Check sheet for the modelled part. Datum: model origin and axes. Units: mm. Face numbers are marked on the shaded views. Give positions to 0.01 mm unless a question says otherwise; leave off trailing zeros. Loops run counter-clockwise (first coordinate to the right, second up) from the corner with the lowest first, then second, coordinate; pieces in that order, holes last. Notation, with made-up numbers: M 30,57 L 49,57 A16 ccw 49,63 Z; hole C 12.5,57 d7. An arc over 180 degrees is marked long. Write each question's results on one line, items separated by ' | '. Start each with the question number.
1. Sectioned sample at B-B on y = 14.25. Record the cut outline in (x, z).
2. Sectioned sample at C-C on x = -14.75. Record the cut outline in (y, z).
3. Go/stop test with flat-tipped pins: pin 1 (2.5 mm diameter, centred on y = 11.88, z = -7, fed in from -X); pin 2 (5 mm diameter, centred on y = 11.88, z = -7, fed in from -X); pin 3 (5 mm diameter, centred on y = 16, z = -4, fed in from +X); pin 4 (4 mm diameter, centred on x = -12, z = -9, fed in from +Y). Record where each tip stops, or that it passes through.
4. Sectioned sample at A-A on x = -9.5. Record the cut outline in (y, z), and give its area (3 significant figures).
5. Material ranges on line 1 along Z through (x, y) = (-15.75, 10.5); line 2 along Y through (x, z) = (-4.45, -7); line 3 along Y through (x, z) = (-14.65, 7), recorded low to high.
6. Draft check along X on the marked faces 1, 2 and 3. Enter one of: pulls with the +X half, pulls with the -X half, needs draft (parallel to the pull), parting line crosses it, or undercut.
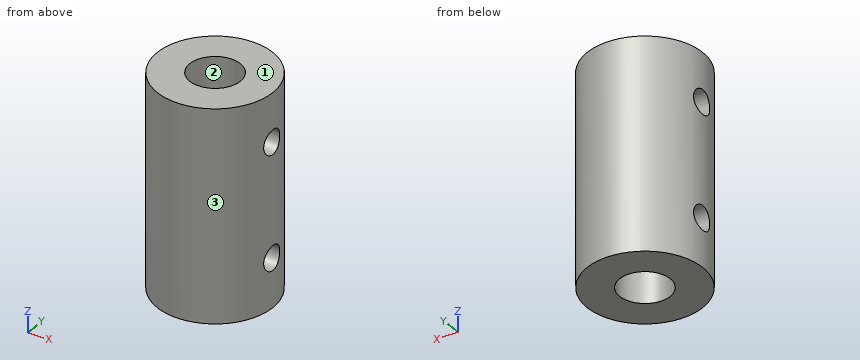
```python
from build123d import *

# Parameters (mm, degrees)
BOSS_EXTRUDE1_DEPTH      = 13
BOSS_EXTRUDE1_DEPTH_BACK = 13
SKETCH1_R                = 7.125
SKETCH1_R_2              = 3.125
SKETCH2_R                = 1.5
CUT_EXTRUDE1_DEPTH       = 20


with BuildPart() as part:
    # Sketch1 → Boss-Extrude1 (new, two sides: drawn at the far end of the back side and taken through both)
    with BuildSketch(Plane.XY.offset(-BOSS_EXTRUDE1_DEPTH_BACK)):
        with Locations((-9.418504592, 11.87550579)):
            Circle(SKETCH1_R)
        with Locations((-9.418504592, 11.87550579)):
            Circle(SKETCH1_R_2, mode=Mode.SUBTRACT)
    extrude(amount=BOSS_EXTRUDE1_DEPTH + BOSS_EXTRUDE1_DEPTH_BACK)

    # Sketch2 → Cut-Extrude1 (cut)
    with BuildSketch(Plane(origin=(0, 0, 0), x_dir=(0, 0, -1), z_dir=(1, 0, 0))):
        with Locations((-7, 11.87550579)):
            Circle(SKETCH2_R)
    cut_extrude1 = extrude(amount=-CUT_EXTRUDE1_DEPTH, mode=Mode.SUBTRACT)

    # Mirror1: Cut-Extrude1 across plane
    add(cut_extrude1.mirror(Plane.XY), mode=Mode.SUBTRACT)


solid = part.part
```
Output values:
1) outline: M -16.14,-13 L -11.45,-13 L -11.45,13 L -16.14,13 Z; M -7.39,-13 L -2.7,-13 L -2.7,13 L -7.39,13 Z
2) outline: M 7.15,-13 L 16.6,-13 L 16.6,13 L 7.15,13 Z; hole C 11.88,-7 d3; hole C 11.88,7 d3
3) pin 1: through | pin 2: x = -16.54 | pin 3: x = -2.48 | pin 4: y = 18.98
4) outline: M 4.75,-13 L 8.75,-13 L 8.75,13 L 4.75,13 Z; M 15,-13 L 19,-13 L 19,13 L 15,13 Z | area: 208 mm2
5) line 1: -13 to -7.6, -6.4 to 6.4, 7.6 to 13 | line 2: 6.77 to 10.38, 13.38 to 16.98 | line 3: 7.04 to 10.38, 13.38 to 16.71
6) face 1: needs draft | face 2: undercut | face 3: parting line crosses it
